Geometry check sheet. Reference: the model listing, model coordinates, mm. Give positions to 0.01 mm unless a question says otherwise; leave off trailing zeros. Put each result on its own line as item: value. Start each with the question number.
```python
from build123d import *

# Parameters (mm, degrees)
SKETCH_1_W          = 40
SKETCH_1_H          = 20
EXTRUDE_1_DEPTH     = 320
SKETCH_2_R          = 2.5
CUT_EXTRUDE_1_DEPTH = 641


with BuildPart() as part:
    # 草图1 → 凸台-拉伸1 (new body, symmetric)
    with BuildSketch(Plane.XY):
        Rectangle(SKETCH_1_W, SKETCH_1_H)
    extrude(amount=EXTRUDE_1_DEPTH, both=True)

    # 草图2 → 切除-拉伸1 (cut, through all)
    with BuildSketch(Plane(origin=(0, 0, -320), x_dir=(-1, 0, 0), z_dir=(0, 0, -1))):
        with Locations((-10, 0)):
            Circle(SKETCH_2_R)
        with Locations((10, 0)):
            Circle(SKETCH_2_R)
        Polygon((-12.5, 10), (-12.5, 9), (-14, 9), (-14, 7.5), (-12, 5.5), (-8, 5.5), (-6, 7.5), (-6, 9), (-7.5, 9), (-7.5, 10), align=None)
        Polygon((-7.5, -9), (-7.5, -10), (-12.5, -10), (-12.5, -9), (-14, -9), (-14, -7.5), (-12, -5.5), (-8, -5.5), (-6, -7.5), (-6, -9), align=None)
        Polygon((-20, 2.5), (-19, 2.5), (-19, 4), (-17.5, 4), (-15.5, 2), (-15.5, -2), (-17.5, -4), (-19, -4), (-19, -2.5), (-20, -2.5), align=None)
        Polygon((7.5, 9), (7.5, 10), (12.5, 10), (12.5, 9), (14, 9), (14, 7.5), (12, 5.5), (8, 5.5), (6, 7.5), (6, 9), align=None)
        Polygon((6, -9), (7.5, -9), (7.5, -10), (12.5, -10), (12.5, -9), (14, -9), (14, -7.5), (12, -5.5), (8, -5.5), (6, -7.5), align=None)
        Polygon((19, -2.5), (20, -2.5), (20, 2.5), (19, 2.5), (19, 4), (17.5, 4), (15.5, 2), (15.5, -2), (17.5, -4), (19, -4), align=None)
    extrude(amount=-CUT_EXTRUDE_1_DEPTH, mode=Mode.SUBTRACT)


solid = part.part
```
Item 1: Gauge pin test, flat ends, axial feed: pin 1 Ø1.2 at (y, z) = (-0.5, 17) entering from -X; pin 2 Ø1.5 at (x, z) = (-9.5, 186.5) entering from -Y. Record the tip position at first contact, or that the pin passes through.
Item 2: Cross-section at A-A (z = -203.5). Count the separate pieces of the cut face and the enclosed holes in it, and give its area (3 significant figures).
Item 3: Thickness scan on line 1 along X through (y, z) = (-7.75, 138); line 2 along X through (y, z) = (2.75, -31.5); line 3 along Y through (x, z) = (10, -112). Record the ranges inside material, lowest first.
Recorded:
1. pin 1: stops at x = -15.5
1. pin 2: stops at y = -5.5
2. separate pieces: 1
2. enclosed holes: 2
2. area: 587 mm^2
3. line 1: x = -20 to -14, -6 to 6, 14 to 20
3. line 2: x = -20 to -19, -16.25 to 16.25, 19 to 20
3. line 3: y = -5.5 to -2.5, 2.5 to 5.5
